Solid Edge part; units mm, degrees
sketch "Sketch1" plane through (0, 0, 0) normal (0, 0, 1) x (1, 0, 0)
  line L0 (-9.5, -30) -> (9.5, -30)
  line L1 (9.5, -30) -> (9.5, 30)
  line L2 (9.5, 30) -> (-9.5, 30)
  line L3 (-9.5, 30) -> (-9.5, -30)
extrude "Protrusion1" add sketch "Sketch1" against normal blind 25
sketch "Sketch2" plane through (0, 0, 0) normal (0, 0, 1) x (-1, 0, 0)
  line L0 (-7.5, -30) -> (7.5, -30)
  line L1 (7.5, -30) -> (7.5, 30)
  line L2 (7.5, 30) -> (-7.5, 30)
  line L3 (-7.5, 30) -> (-7.5, -30)
extrude "ExtrudedCutout_1" cut sketch "Sketch2" along normal mid plane 109.0944
sketch "Sketch3" plane through (9.5, 0, -12.5) normal (1, 0, 0) x (0, 1, 0)
  line L0 (-30, 10.5) -> (30, 10.5)
  line L1 (30, 10.5) -> (30, 12.5)
  line L2 (30, 12.5) -> (-30, 12.5)
  line L3 (-30, 12.5) -> (-30, 10.5)
extrude "ExtrudedProtrusion_2" add sketch "Sketch3" along normal blind 8
sketch "Sketch4" plane through (-9.5, 0, -12.5) normal (-1, 0, 0) x (0, -1, 0)
  line L0 (-30, 12.5) -> (30, 12.5)
  line L1 (30, 12.5) -> (30, 10.5)
  line L2 (30, 10.5) -> (-30, 10.5)
  line L3 (-30, 10.5) -> (-30, 12.5)
extrude "ExtrudedProtrusion_3" add sketch "Sketch4" along normal blind 8
sketch "Sketch5" plane through (-7.5, 0, -12.5) normal (1, 0, 0) x (0, 1, 0)
  line L0 (30, -2.5) -> (-30, 12.5)
  line L1 (-30, 12.5) -> (-30, -12.5)
  line L2 (-30, -12.5) -> (30, -12.5)
  line L3 (30, -12.5) -> (30, -2.5)
extrude "Protrusion2" add sketch "Sketch5" along normal blind 15
sketch "Sketch6" plane through (9.5, 0, -13.5) normal (1, 0, 0) x (0, 1, 0)
  line L0 (30, -3.5) -> (-30, -3.5)
  line L1 (-30, -3.5) -> (-30, -11.5)
  line L2 (-30, -11.5) -> (30, -11.5)
  line L3 (30, -11.5) -> (30, -3.5)
extrude "ExtrudedCutout_2" cut sketch "Sketch6" along normal mid plane 141.9201
sketch "Sketch7" plane through (9.5, 0, -9.5) normal (1, 0, 0) x (0, 1, 0)
  line L0 (-30, 7.5) -> (30, -7.5)
  line L1 (30, -7.5) -> (-30, -7.5)
  line L2 (-30, -7.5) -> (-30, 7.5)
extrude "ExtrudedCutout_3" cut sketch "Sketch7" along normal mid plane 158.0788
The listing builds one solid part. Answer for the finished solid, in the listing's coordinates (mm). A direction names the side the tool comes from. Give positions to 0.01 mm unless a question says otherwise; leave off trailing zeros. Order: outer loops, then holes, each group sorted by start corner. A loop starts at its lowest first (then second) coordinate and runs counter-clockwise, first axis right, second up. Notation, with made-up numbers: M 7.5,42 L 61.5,42 A11 ccw 61.5,54 Z; hole C 73.25,51 d8. An arc over 180 degrees is marked long. Put each result on its own line as item: value. Start each with the question number.
Item 1: The part is cut by section B-B, the plane y = -26. Determine the outline of the cut face in (x, z), and give its area (3 significant figures).
Item 2: The part is cut by section A-A, the plane z = -12.75. Determine the outline of the cut face in (x, y).
Item 3: Which of the six approach directions +Z, -Z, +X, -X, +Y, -Y give full straight-line access (tool end or side, diameter ignored) to faces 5 (the face through (13, 0, -2)), 6 (the face through (-1.2, 30, -15.4)), 7 (the face through (7.5, 13, -4)), 8 (the face through (-13, 0, -2))?
Item 4: Flat-ended cylindrical pins translate along their axes: P1, Ø3, axis at x = 0, y = -0.5, coming from the +Z side; P2, Ø2, axis at x = -2.5, y = 6, coming from the -Z side; P3, Ø5, axis at x = -3, y = 17, coming from the +Z side (3 decimals). Find the tip coordinate at first contact, or state that the pin passes through.
Item 5: For a pull along X with two mould halves and no side action, classify faces 1 (the face through (17.5, 0, -1)), 2 (the face through (-7.5, 14, -4)), 3 (the face through (-9.5, 7, -8)), 4 (the face through (-0.1, 0.4, -7.6)) as +X half, -X half, draft (parallel to the pull), parting line (faces both ways), or undercut.
Item 6: Find the intervals of material crossed by line 1 along X through (y, z) = (12, -1.75); line 2 along X through (y, z) = (25, -6.5); line 3 along Z through (x, y) = (-15.5, 21), in increasing order.
Item 7: The part is cut by section D-D, the plane z = -8.25. Determine the outline of the cut face in (x, y), and give its area (3 significant figures).
Item 8: The part is cut by section C-C, the plane y = 20. Determine the outline of the cut face in (x, z), and give its area (3 significant figures).
Answer key:
1. outline: M -17.5,-2 L -9.5,-2 L -9.5,-3 L 9.5,-3 L 9.5,-2 L 17.5,-2 L 17.5,0 L 7.5,0 L 7.5,-1 L -7.5,-1 L -7.5,0 L -17.5,0 Z
1. area: 74.0 mm²
2. outline: M -9.5,13 L 9.5,13 L 9.5,30 L 7.5,30 L 7.5,21 L -7.5,21 L -7.5,30 L -9.5,30 Z
3. face 5: -Z, +X, +Y, -Y
3. face 6: +Z, -Z, +X, -X, +Y
3. face 7: +Z, +Y
3. face 8: -Z, -X, +Y, -Y
4. P1: stops at z = -7
4. P2: stops at z = -11.25
4. P3: stops at z = -11.125
5. face 1: +X half
5. face 2: undercut
5. face 3: -X half
5. face 4: undercut
6. line 1: x = -17.5 to -7.5, 7.5 to 17.5
6. line 2: x = -9.5 to -7.5, 7.5 to 9.5
6. line 3: z = -2 to 0
7. outline: M -9.5,-5 L 9.5,-5 L 9.5,30 L 7.5,30 L 7.5,3 L -7.5,3 L -7.5,30 L -9.5,30 Z
7. area: 260 mm²
8. outline: M -17.5,-2 L -9.5,-2 L -9.5,-14.5 L 9.5,-14.5 L 9.5,-2 L 17.5,-2 L 17.5,0 L 7.5,0 L 7.5,-12.5 L -7.5,-12.5 L -7.5,0 L -17.5,0 Z
8. area: 120 mm²
